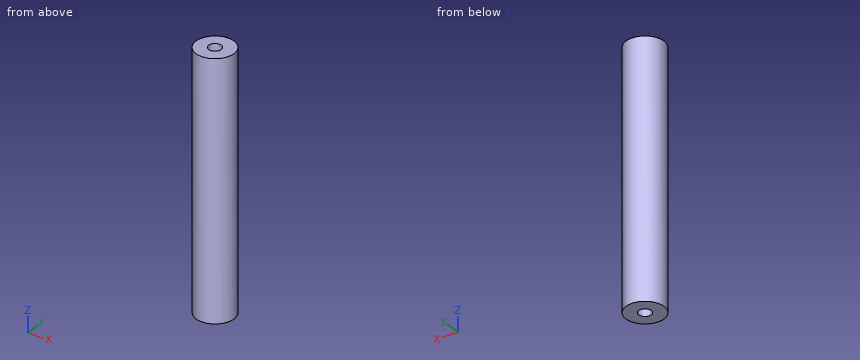
```python
from build123d import *

# Parameters (mm, degrees)
SKETCH1_R           = 4.7625
BOSS_EXTRUDE2_DEPTH = 63.5
SKETCH5_R           = 1.5875
CUT_EXTRUDE1_DEPTH  = 12.7
CUT_EXTRUDE2_START  = 12.7
SKETCH6_R           = 1.5875
CUT_EXTRUDE2_DEPTH  = 12.7


with BuildPart() as part:
    # Sketch1 → Boss-Extrude2 (new body)
    with BuildSketch(Plane.XY):
        Circle(SKETCH1_R)
    extrude(amount=BOSS_EXTRUDE2_DEPTH)

    # Sketch5 → Cut-Extrude1 (cut)
    with BuildSketch(Plane.XY):
        Circle(SKETCH5_R)
    extrude(amount=CUT_EXTRUDE1_DEPTH, mode=Mode.SUBTRACT)

    # Sketch6 → Cut-Extrude2 (cut)
    with BuildSketch(Plane(origin=(0, 0, 63.5), x_dir=(-1, 0, 0), z_dir=(0, 0, -1)).offset(CUT_EXTRUDE2_START)):
        with Locations(Location((0, 0, 0), (0, 0, 180))):
            Circle(SKETCH6_R)
    extrude(amount=-CUT_EXTRUDE2_DEPTH, mode=Mode.SUBTRACT)


solid = part.part
```
For this review, take the finished solid that the model builds, in its own axes (mm). Coordinates: 2 decimals unless noted, no trailing zeros. Write each loop counter-clockwise with the first axis right and the second up, starting at its lowest first coordinate (ties: lowest second). Pieces come first, ordered by that corner, then holes.
(1) Add section D-D on z = 27. Give the boundary of the cut face in (x, y) (1 decimal), then the cut area to 3 significant figures.
(2) Wall thickness on probe 1 along Y at (x, z) = (0, 9); probe 2 along Y at (x, z) = (1, 8.5); probe 3 along Z at (x, y) = (0.25, 0.75): over which ranges is each line inside the solid? List them lowest first.
(3) Add section A-A on x = 0. Give the boundary of the cut face in (y, z).
(4) For pin 1 Ø2 at (x, z) = (-1.5, 16.5) entering from +Y; pin 2 Ø1 at (x, y) = (0.5, 0) entering from -Z; pin 3 Ø1.5 at (y, z) = (-2, 31) entering from -X, all flat-tipped, find the tip position at first contact; note any pin that passes through.
(5) Add section C-C on z = 10.5. Give the boundary of the cut face in (x, y) (1 decimal).
Answer sheet:
1. outline: circle Ø9.5 at (0, 0)
1. area: 71.3 mm2
2. probe 1: y = -4.76 to -1.59, 1.59 to 4.76
2. probe 2: y = -4.66 to -1.23, 1.23 to 4.66
2. probe 3: z = 12.7 to 50.8
3. outline: (-4.76, 0) - (-1.59, 0) - (-1.59, 12.7) - (1.59, 12.7) - (1.59, 0) - (4.76, 0) - (4.76, 63.5) - (1.59, 63.5) - (1.59, 50.8) - (-1.59, 50.8) - (-1.59, 63.5) - (-4.76, 63.5) - close
4. pin 1: stops at y = 4.74
4. pin 2: stops at z = 12.7
4. pin 3: stops at x = -4.6
5. outline: circle Ø9.5 at (0, 0); hole circle Ø3.2 at (0, 0)
